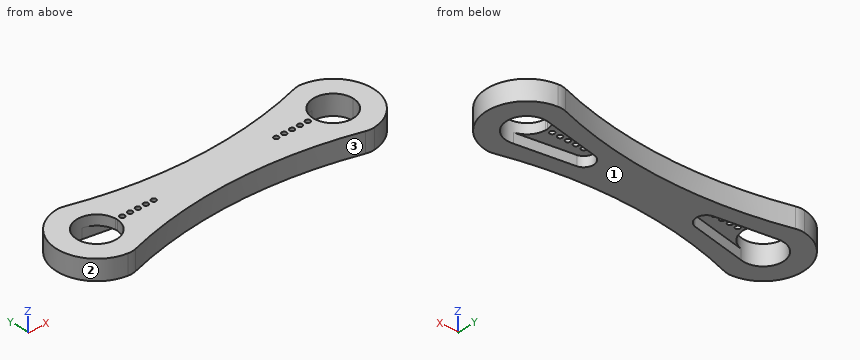
from build123d import *

# Parameters (mm, degrees)
SKETCH1_R           = 5
BOSS_EXTRUDE1_DEPTH = 5
FILLET1_R           = 5
SKETCH2_R           = 0.6
CUT_EXTRUDE1_DEPTH  = 5
SKETCH3_R           = 0.6
CUT_EXTRUDE2_DEPTH  = 2.5


with BuildPart() as part:
    # Sketch1 → Boss-Extrude1 (new body)
    with BuildSketch(Plane.XY):
        with BuildLine():
            ThreePointArc((0, 10), (-10, 0), (0, -10))
            ThreePointArc((0, -10), (30, -5.393920142), (60, -10))
            ThreePointArc((60, -10), (70, 0), (60, 10))
            ThreePointArc((60, 10), (30, 5.393920142), (0, 10))
        make_face()
        Circle(SKETCH1_R, mode=Mode.SUBTRACT)
        with Locations((60, 0)):
            Circle(SKETCH1_R, mode=Mode.SUBTRACT)
    extrude(amount=BOSS_EXTRUDE1_DEPTH)

    # Fillet1
    fillet1_edges = [part.edges().sort_by_distance(p)[0] for p in [
        (60, 10, 2.5),
        (60, -10, 2.5),
        (0, -10, 2.5),
        (0, 10, 2.5),
    ]]
    fillet(fillet1_edges, radius=FILLET1_R)

    # Sketch2 → Cut-Extrude1 (cut)
    with BuildSketch(Plane(origin=(0, 0, 0), x_dir=(-1, 0, 0), z_dir=(0, 0, -1))):
        with Locations((-4.45, 0)):
            Circle(SKETCH2_R)
        with Locations((-6.45, 0)):
            Circle(SKETCH2_R)
        with Locations((-8.45, 0)):
            Circle(SKETCH2_R)
        with Locations((-10.45, 0)):
            Circle(SKETCH2_R)
        with Locations((-12.45, 0)):
            Circle(SKETCH2_R)
        with Locations((-14.45, 0)):
            Circle(SKETCH2_R)
    cut_extrude1 = extrude(amount=-CUT_EXTRUDE1_DEPTH, mode=Mode.SUBTRACT)

    # Sketch3 → Cut-Extrude2 (cut)
    with BuildSketch(Plane(origin=(0, 0, 0), x_dir=(-1, 0, 0), z_dir=(0, 0, -1))):
        with BuildLine():
            Line((-15.012283737, -2.435946838), (-1.124567474, -4.871893677))
            ThreePointArc((-1.124567474, -4.871893677), (-3.832599709, -3.211102532), (-4.993539326, -0.254096441))
            ThreePointArc((-4.993539326, -0.254096441), (-5.05, 0), (-4.993539326, 0.254096441))
            ThreePointArc((-4.993539326, 0.254096441), (-3.746221254, 3.311468906), (-0.865051903, 4.924600005))
            Line((-0.865051903, 4.924600005), (-14.882525952, 2.462300002))
            ThreePointArc((-14.882525952, 2.462300002), (-16.949123268, 0.066203422), (-15.012283737, -2.435946838))
        make_face()
        with Locations((-12.45, 0)):
            Circle(SKETCH3_R, mode=Mode.SUBTRACT)
        with Locations((-6.45, 0)):
            Circle(SKETCH3_R, mode=Mode.SUBTRACT)
        with Locations((-8.45, 0)):
            Circle(SKETCH3_R, mode=Mode.SUBTRACT)
        with Locations((-10.45, 0)):
            Circle(SKETCH3_R, mode=Mode.SUBTRACT)
        with Locations((-14.45, 0)):
            Circle(SKETCH3_R, mode=Mode.SUBTRACT)
    cut_extrude2 = extrude(amount=-CUT_EXTRUDE2_DEPTH, mode=Mode.SUBTRACT)

    # Mirror2: Cut-Extrude1, Cut-Extrude2 across plane
    add(cut_extrude1.mirror(Plane(origin=(30, 0, 0), x_dir=(0, 0, 1), z_dir=(1, 0, 0))), mode=Mode.SUBTRACT)
    add(cut_extrude2.mirror(Plane(origin=(30, 0, 0), x_dir=(0, 0, 1), z_dir=(1, 0, 0))), mode=Mode.SUBTRACT)


solid = part.part
Here's how the part is built. I have some questions about the finished solid (model axes, mm). Face numbers are marked on the shaded views. Round coordinates to 2 decimals unless told otherwise and drop trailing zeros. Loops run counter-clockwise (first coordinate to the right, second up) from the corner with the lowest first, then second, coordinate; pieces in that order, holes last. Notation, with made-up numbers: (66, 48) -> (107, 48) arc R14 ccw to (107, 73) -> close; hole circle Ø11 at (65.5, 65). An arc over 180 degrees is marked (long way). Write each question's results on one line, items separated by ' | '.
(1) If we section it at A-A, the plane x = 58: List the corners of the cut face in (y, z) for me.
Worked answers:
outline: (-9.39, 0) -> (-4.72, 0) -> (-4.72, 2.5) -> (-4.58, 2.5) -> (-4.58, 5) -> (-9.39, 5) -> close; (4.58, 2.5) -> (4.73, 2.5) -> (4.73, 0) -> (9.39, 0) -> (9.39, 5) -> (4.58, 5) -> close
(2) If we section it at D-D, the plane y = -3.5: List the corners of the cut face in (x, z) for me.
Worked answers:
outline: (-9.37, 0) -> (-3.57, 0) -> (-3.57, 5) -> (-9.37, 5) -> close; (3.57, 2.5) -> (8.95, 2.5) -> (8.95, 0) -> (51.05, 0) -> (51.05, 2.5) -> (56.43, 2.5) -> (56.43, 5) -> (3.57, 5) -> close; (63.57, 0) -> (69.37, 0) -> (69.37, 5) -> (63.57, 5) -> close
(3) If we section it at B-B, the plane y = -8.5: List the corners of the cut face in (x, z) for me, then the cut area to 3 significant figures.
Worked answers:
outline: (-5.27, 0) -> (5.27, 0) -> (5.27, 5) -> (-5.27, 5) -> close; (54.73, 0) -> (65.27, 0) -> (65.27, 5) -> (54.73, 5) -> close | area: 105 mm2
(4) We'd pull the mould along X, two halves only. Please class the marked faces 1, 2 and 3: released by +X, released by -X, zero draft, split by the parting line, or undercut.
Worked answers:
face 1: zero draft | face 2: released by -X | face 3: undercut
(5) For P1, Ø1.6, axis at x = 47.55, y = 0, coming from the -Z side; P2, Ø3, axis at x = 10, z = 3.5, coming from the +Y side, each with a flat end and sliding along its axis, tell me the tip position at first contact or that it passes through.
Worked answers:
P1: z = 2.5 | P2: y = 7.73
(6) If we section it at C-C, the plane z = 3.7: Give the number of separate pieces and of enclosed holes in the cut face, then the cut area to 3 significant figures.
Worked answers:
separate pieces: 1 | enclosed holes: 12 | area: 975 mm2
(7) If I drill on L1, parallel to X at y = -1.25, z = 3.3; L2, parallel to Y at x = 60, z = 4.45; L3, parallel to Y at x = 6, z = 1.1, over which ranges is the centre line in solid material (lowest first)?
Worked answers:
L1: -9.92 to -4.84, 4.84 to 55.16, 64.84 to 69.92 | L2: -9.92 to -5, 5 to 9.92 | L3: -8.32 to -4.02, 4.02 to 8.32
